Print and shaded views of the part. All mm, measured from the part's lowest x, y and z. A direction names the side the tool comes from. Give positions to 0.01 mm unless a question says otherwise; leave off trailing zeros. Write each loop counter-clockwise with the first axis right and the second up, starting at its lowest first coordinate (ties: lowest second). Pieces come first, ordered by that corner, then holes. Notation, with made-up numbers: (24.25, 40.5) -> (56.25, 40.5) arc R26 cw to (56.25, 68.5) -> close; hole circle Ø1 at (85.25, -15.5). An arc over 180 degrees is marked (long way). Put each result on its own line as item: value.
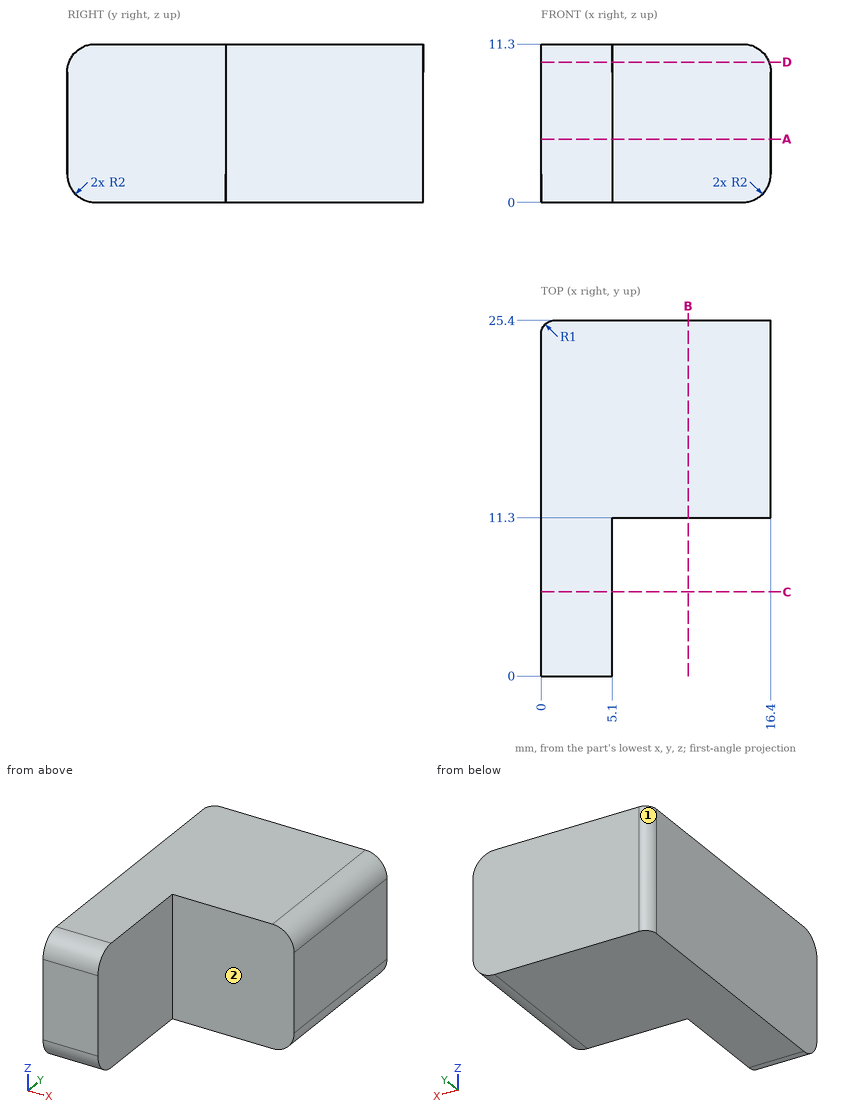
1) Slice it at A-A (z = 4.5). Write the cut outline in (x, y), plus the area to 3 significant figures.
Filled sheet:
outline: (0, 0) -> (5.1, 0) -> (5.1, 11.3) -> (16.4, 11.3) -> (16.4, 25.4) -> (1, 25.4) arc R1 ccw to (0, 24.4) -> close
area: 289 mm2
2) Slice it at B-B (x = 10.5). Write the cut outline in (y, z), plus the area to 3 significant figures.
Filled sheet:
outline: (11.3, 0) -> (25.4, 0) -> (25.4, 11.3) -> (11.3, 11.3) -> close
area: 159 mm2
3) Slice it at C-C (y = 6). Write the cut outline in (x, z), plus the area to 3 significant figures.
Filled sheet:
outline: (0, 0) -> (5.1, 0) -> (5.1, 11.3) -> (0, 11.3) -> close
area: 57.6 mm2
4) Tool access for the marked faces 1 and 2: list every direction of +Z, -Z, +X, -X, +Y, -Y with a clear straight run to the whole face (end or side of a thin tool).
Filled sheet:
face 1: +Z, -Z, -X, +Y
face 2: +Z, -Z, +X, -Y
5) Slice it at D-D (z = 10). Write the cut outline in (x, y).
Filled sheet:
outline: (0, 0.13) -> (5.1, 0.13) -> (5.1, 11.3) -> (16.27, 11.3) -> (16.27, 25.4) -> (1, 25.4) arc R1 ccw to (0, 24.4) -> close
6) Wall check: L1, parallel to Y at x = 12.5, z = 8.75; L2, parallel to X at y = 2.25, z = 9; L3, parallel to Z at x = 14.5, y = 11.5. Give the ranges that are in metal, low to high.
Filled sheet:
L1: 11.3 to 25.4
L2: 0 to 5.1
L3: 0 to 11.3
7) Pin check, flat tips, straight feed: pin 1 (3.5 mm diameter, centred on y = 3.5, z = 7.5, fed in from +X); pin 2 (1 mm diameter, centred on x = 8.5, z = 5, fed in from -Y). Stop position of each tip, or through.
Filled sheet:
pin 1: x = 5.1
pin 2: y = 11.3
